```python
from build123d import *

# Parameters (mm, degrees)
F1_DEPTH = 4
F3_DEPTH = 2.5
F5_DEPTH = 2
F7_DEPTH = 5.6
F9_DEPTH = 25


with BuildPart() as f1:
    # F0 (on Top) → F1 (new body)
    with BuildSketch(Plane.XY):
        with BuildLine():
            Line((3.8369910086, 2.8), (-3.8369910086, 2.8))
            ThreePointArc((-3.8369910086, 2.8), (-4.75, 0), (-3.8369910086, -2.8))
            Line((-3.8369910086, -2.8), (3.8369910086, -2.8))
            ThreePointArc((3.8369910086, -2.8), (4.75, 0), (3.8369910086, 2.8))
        make_face()
    extrude(amount=F1_DEPTH)

    # F2 (on face) → F3 (join)
    with BuildSketch(Plane(origin=(0, 0, 0), x_dir=(1, 0, 0), z_dir=(0, 0, -1))):
        with BuildLine():
            ThreePointArc((1.0770329614, -2.8), (2.4729636961, -1.6983670268), (3, 0))
            ThreePointArc((3, 0), (2.4729636961, 1.6983670268), (1.0770329614, 2.8))
            Line((1.0770329614, 2.8), (-1.0770329614, 2.8))
            ThreePointArc((-1.0770329614, 2.8), (-3, 0), (-1.0770329614, -2.8))
            Line((-1.0770329614, -2.8), (1.0770329614, -2.8))
        make_face()
    extrude(amount=F3_DEPTH)

    # F4 (on face) → F5 (join)
    with BuildSketch(Plane(origin=(0, 0, -2.5), x_dir=(1, 0, 0), z_dir=(0, 0, -1))):
        with BuildLine():
            ThreePointArc((3.8369910086, -2.8), (4.75, 0), (3.8369910086, 2.8))
            Line((3.8369910086, 2.8), (1.0770329614, 2.8))
            Line((1.0770329614, 2.8), (-1.0770329614, 2.8))
            Line((-1.0770329614, 2.8), (-3.8369910086, 2.8))
            ThreePointArc((-3.8369910086, 2.8), (-4.75, 0), (-3.8369910086, -2.8))
            Line((-3.8369910086, -2.8), (-1.0770329614, -2.8))
            Line((-1.0770329614, -2.8), (1.0770329614, -2.8))
            Line((1.0770329614, -2.8), (3.8369910086, -2.8))
        make_face()
    extrude(amount=F5_DEPTH)

    # F6 (on face) → F7 (join)
    with BuildSketch(Plane.XZ.offset(2.8)):
        with BuildLine():
            ThreePointArc((0, -4.5), (3.00520382, -5.74479618), (4.25, -8.75))
            ThreePointArc((4.25, -8.75), (4.0532970407, -10.0279996479), (3.4813961882, -11.1876998545))
            Line((3.4813961882, -11.1876998545), (4.3005482325, -11.7612762908))
            ThreePointArc((4.3005482325, -11.7612762908), (5.0070139914, -10.3287054474), (5.25, -8.75))
            ThreePointArc((5.25, -8.75), (4.6767556467, -6.3645322008), (3.0822070015, -4.5))
            Line((3.0822070015, -4.5), (0, -4.5))
        make_face()
        with BuildLine():
            ThreePointArc((-3.4813961882, -11.1876998545), (-3.769796041, -6.7875683938), (0, -4.5))
            Line((0, -4.5), (-3.0822070015, -4.5))
            ThreePointArc((-3.0822070015, -4.5), (-5.1776251365, -7.8812664702), (-4.3005482325, -11.7612762908))
            Line((-4.3005482325, -11.7612762908), (-3.4813961882, -11.1876998545))
        make_face()
    extrude(amount=-F7_DEPTH)

    # F8 (on face) → F9 (cut)
    with BuildSketch(Plane(origin=(0, 2.8, 0), x_dir=(-1, 0, 0), z_dir=(0, 1, 0))):
        Polygon((4.75, 2), (4.75, 4), (3.8369910086, 4), (3.8369910086, 2.9130089914), align=None)
        Polygon((3.8369910086, 2.9130089914), (3.8369910086, 4), (2.75, 4), align=None)
        Polygon((-3.8369910086, 2.9130089914), (-2.75, 4), (-3.8369910086, 4), align=None)
        Polygon((-3.8369910086, 2.9130089914), (-3.8369910086, 4), (-4.75, 4), (-4.75, 2), align=None)
    extrude(amount=-F9_DEPTH, mode=Mode.SUBTRACT)


solid = f1.part
```
Here's how the part is built. I have some questions about the finished solid (model axes, mm). A direction names the side the tool comes from. Round coordinates to 2 decimals unless told otherwise and drop trailing zeros. Loops run counter-clockwise (first coordinate to the right, second up) from the corner with the lowest first, then second, coordinate; pieces in that order, holes last. Notation, with made-up numbers: (65, 42.25) -> (102, 42.25) arc R17 cw to (102, 74.25) -> close; hole circle Ø9 at (73.25, 60). An arc over 180 degrees is marked (long way). Answer as CSV lines item,"result". Start each with the question number.
1. Imagine slicing it at B-B on x = 2. Write out the boundary of the cut face in (y, z), plus the area to 3 significant figures.
2. Imagine slicing it at A-A on z = -10. Write out the boundary of the cut face in (x, y).
3. I'm going to push flat-ended pins straight in: P1, Ø2, axis at y = -1.5, z = -4.5, coming from the +X side; P2, Ø2, axis at x = 3, y = 0, coming from the -Z side; P3, Ø1.1, axis at x = -2, y = 0, coming from the -Z side. Where does each tip first touch, or does it pass through?
4. If we mould it in two halves opening along Z, with no side actions, what happens to faces 1 (the face through (4.75, 0.04, -3.49)), 2 (the face through (-4, 0, -4.5)), 3 (the face through (0, 0, 4)), 4 (the face through (-3.3, 0, 0))? For each: pulls with the +Z half, pulls with the -Z half, needs draft (parallel to the pull), parting line crosses it, or undercut.
5. Imagine slicing it at D-D on z = -2. Write out the boundary of the cut face in (x, y).
6. For faces 5 (the face through (-3.9, -0.04, -11.48)), 6 (the face through (-3, 0, -1)), 7 (the face through (4.75, -0.04, 1.11)), 8 (the face through (-4.75, 0.04, 1.11)), 9 (the face through (3.3, 0, -2.5)), which set-ups out of +Z, -Z, +X, -X, +Y, -Y let a thin tool reach every point of the face, with its end or its side?
7. Imagine slicing it at C-C on y = 1.2. Write out the boundary of the cut face in (x, z), plus the area to 3 significant figures.
8. I need wall thicknesses on probe 1 along X at (y, z) = (-0.1, -1); probe 2 along X at (y, z) = (0.25, -8); probe 3 along X at (y, z) = (0.7, -7). Which ranges of each line are inside material? Lowest first, please. Write a range as from..to.
Solution:
1,outline,"(-2.8, -5) -> (2.8, -5) -> (2.8, -2.5) -> (2.24, -2.5) -> (2.24, 0) -> (2.8, 0) -> (2.8, 4) -> (-2.8, 4) -> (-2.8, 0) -> (-2.24, 0) -> (-2.24, -2.5) -> (-2.8, -2.5) -> close"
1,area,"47.6 mm²"
2,outline,"(-5.1, -2.8) -> (-4.06, -2.8) -> (-4.06, 2.8) -> (-5.1, 2.8) -> close; (4.06, -2.8) -> (5.1, -2.8) -> (5.1, 2.8) -> (4.06, 2.8) -> close"
3,P1,"x = 4.72"
3,P2,"z = -11.55"
3,P3,"z = -5.35"
4,face 1,"needs draft"
4,face 2,"undercut"
4,face 3,"pulls with the +Z half"
4,face 4,"undercut"
5,outline,"(-1.08, -2.8) -> (1.08, -2.8) arc R3 ccw to (1.08, 2.8) -> (-1.08, 2.8) arc R3 ccw to start"
6,face 5,"-Z, +Y, -Y"
6,face 6,"-X"
6,face 7,"+Z, +X"
6,face 8,"+Z, -X"
6,face 9,"+X"
7,outline,"(-4.6, -4.5) -> (-3.08, -4.5) arc R5.25 ccw to (-4.3, -11.76) -> (-3.48, -11.19) arc R4.25 cw (long way) to (3.48, -11.19) -> (4.3, -11.76) arc R5.25 ccw to (3.08, -4.5) -> (4.6, -4.5) -> (4.6, -2.5) -> (2.75, -2.5) -> (2.75, 0) -> (4.6, 0) -> (4.6, 2.15) -> (2.75, 4) -> (-2.75, 4) -> (-4.6, 2.15) -> (-4.6, 0) -> (-2.75, 0) -> (-2.75, -2.5) -> (-4.6, -2.5) -> close"
7,area,"82.0 mm²"
8,probe 1,"-3..3"
8,probe 2,"-5.2..-4.18, 4.18..5.2"
8,probe 3,"-4.95..-3.87, 3.87..4.95"
